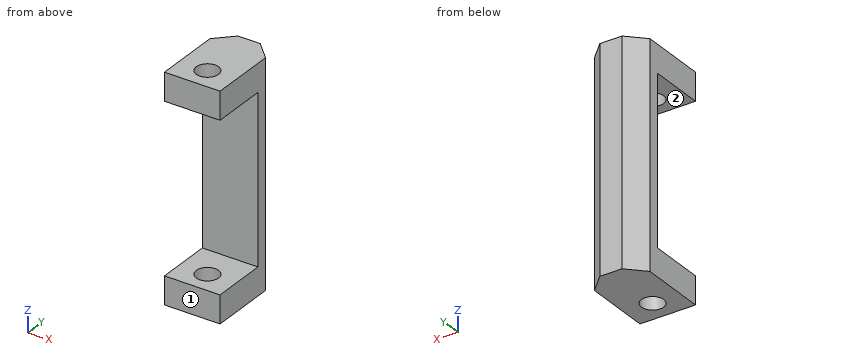
```python
from build123d import *

# Parameters (mm, degrees)
BOSS_EXTRUDE1_DEPTH         = 12.7
TAP_DRILL_FOR_1_4_20_TAP1_D = 5.1054
CHAMFER1_SIZE               = 3.81


with BuildPart() as part:
    # Sketch1 → Boss-Extrude1 (new body)
    with BuildSketch(Plane(origin=(0, 0, 0), x_dir=(0, 0, -1), z_dir=(1, 0, 0))):
        Polygon((25.4, 0), (-25.4, 0), (-25.4, -19.05), (-19.05, -19.05), (-19.05, -6.35), (19.05, -6.35), (19.05, -19.05), (25.4, -19.05), align=None)
    extrude(amount=BOSS_EXTRUDE1_DEPTH)

    # Tap Drill for 1/4-20 Tap1 (through all)
    with Locations(Plane(origin=(6.35, -13.97, -25.4), x_dir=(-1, 0, 0), z_dir=(0, 0, -1))):
        with Locations((0, 0)):
            Hole(TAP_DRILL_FOR_1_4_20_TAP1_D / 2)

    # Chamfer1
    chamfer1_edges = [part.edges().sort_by_distance(p)[0] for p in [
        (12.7, 0, 0),
        (0, 0, 0),
    ]]
    chamfer(chamfer1_edges, length=CHAMFER1_SIZE)


solid = part.part
```
Here's how the part is built. I have some questions about the finished solid (model axes, mm). Face numbers are marked on the shaded views. A direction names the side the tool comes from. Coordinates: 2 decimals unless noted, no trailing zeros. Order: outer loops, then holes, each group sorted by start corner. A loop starts at its lowest first (then second) coordinate and runs counter-clockwise, first axis right, second up. Notation, with made-up numbers: M 26,-31 L 39,-31 A20 cw 39,-5 Z; hole C -7.75,51 d3. An arc over 180 degrees is marked long. Answer as a JSON object with one key per item and string values. Group by question number.
(1) Suppose I cut it at A-A, the plane x = 6.35. Please give me the cut outline in (y, z).
(2) Suppose I cut it at D-D, the plane x = 2.5. Please give me the cut outline in (y, z), then the cut area to 3 significant figures.
(3) Suppose I cut it at C-C, the plane y = -13.97. Please give me the cut outline in (x, z).
(4) Which directions (+Z, -Z, +X, -X, +Y, -Y) give clear straight access to the entire face, cutting with the end or side of a thin tool? Please do the marked faces 1 and 2.
(5) Suppose I cut it at B-B, the plane z = 20.5. Please give me the cut outline in (x, y), then the cut area to 3 significant figures.
(6) For pin 1 (8 mm diameter, centred on y = -2.5, z = 7, fed in from +X); pin 2 (2 mm diameter, centred on x = 3, z = -16, fed in from -Y); pin 3 (4.5 mm diameter, centred on x = 6.35, y = -13.97, fed in from +Z), each with a flat end and sliding along its axis, tell me the tip position at first contact or that it passes through.
(7) I need wall thicknesses on probe 1 along Y at (x, z) = (6.35, 20.5); probe 2 along Z at (x, y) = (4.25, -17.75); probe 3 along Y at (x, z) = (5.25, 8.5). Which ranges of each line are inside material? Lowest first, please.
Values found:
{
 "1": {"outline": "M -19.05,-25.4 L -16.52,-25.4 L -16.52,-19.05 L -19.05,-19.05 Z; M -19.05,19.05 L -16.52,19.05 L -16.52,25.4 L -19.05,25.4 Z; M -11.42,-25.4 L 0,-25.4 L 0,25.4 L -11.42,25.4 L -11.42,19.05 L -6.35,19.05 L -6.35,-19.05 L -11.42,-19.05 Z"},
 "2": {"outline": "M -19.05,-25.4 L -1.31,-25.4 L -1.31,25.4 L -19.05,25.4 L -19.05,19.05 L -6.35,19.05 L -6.35,-19.05 L -19.05,-19.05 Z", "area": "417 mm^2"},
 "3": {"outline": "M 0,-25.4 L 3.8,-25.4 L 3.8,-19.05 L 0,-19.05 Z; M 0,19.05 L 3.8,19.05 L 3.8,25.4 L 0,25.4 Z; M 8.9,-25.4 L 12.7,-25.4 L 12.7,-19.05 L 8.9,-19.05 Z; M 8.9,19.05 L 12.7,19.05 L 12.7,25.4 L 8.9,25.4 Z"},
 "4": {"face 1": "+Z, -Z, +X, -X, -Y", "face 2": "+X, -X, -Y"},
 "5": {"outline": "M 0,-19.05 L 12.7,-19.05 L 12.7,-3.81 L 8.89,0 L 3.81,0 L 0,-3.81 Z; hole C 6.35,-13.97 d5.11", "area": "207 mm^2"},
 "6": {"pin 1": "stops at x = 12.7", "pin 2": "stops at y = -6.35", "pin 3": "passes through"},
 "7": {"probe 1": "y = -19.05 to -16.52, -11.42 to 0", "probe 2": "z = -25.4 to -19.05, 19.05 to 25.4", "probe 3": "y = -6.35 to 0"}
}
